```python
from build123d import *

# Parameters (mm, degrees)
SKETCH1_W           = 40.64
SKETCH1_H           = 40.64
BOSS_EXTRUDE1_DEPTH = 5
CUT_EXTRUDE1_REACH  = 7
SKETCH2_R           = 3.085
CHAMFER1_SIZE       = 2.5
SKETCH3_R           = 11.5
CUT_EXTRUDE2_DEPTH  = 1.6
SKETCH7_R           = 0.8
CUT_EXTRUDE6_DEPTH  = 4.4
CUT_EXTRUDE7_DEPTH  = 1.6


with BuildPart() as part:
    # Sketch1 → Boss-Extrude1 (new body)
    with BuildSketch(Plane(origin=(0, 0, 0), x_dir=(1, 0, 0), z_dir=(0, 1, 0))):
        Rectangle(SKETCH1_W, SKETCH1_H)
    extrude(amount=BOSS_EXTRUDE1_DEPTH)

    # Sketch2 → Cut-Extrude1 (cut, up to next)
    with BuildSketch(Plane(origin=(0, 5, 0), x_dir=(1, 0, 0), z_dir=(0, 1, 0)), mode=Mode.PRIVATE) as cut_extrude1_sk1:
        with Locations((-15, 15)):
            Circle(SKETCH2_R)
    cut_extrude1_tool1 = extrude(cut_extrude1_sk1.sketch, amount=-CUT_EXTRUDE1_REACH, mode=Mode.PRIVATE) & part.part
    add(cut_extrude1_tool1.solids().sort_by_distance((-15, 5, -15))[0], mode=Mode.SUBTRACT)
    # Sketch2 → Cut-Extrude1 (cut, up to next)
    with BuildSketch(Plane(origin=(0, 5, 0), x_dir=(1, 0, 0), z_dir=(0, 1, 0)), mode=Mode.PRIVATE) as cut_extrude1_sk2:
        with Locations((15, 15)):
            Circle(SKETCH2_R)
    cut_extrude1_tool2 = extrude(cut_extrude1_sk2.sketch, amount=-CUT_EXTRUDE1_REACH, mode=Mode.PRIVATE) & part.part
    add(cut_extrude1_tool2.solids().sort_by_distance((15, 5, -15))[0], mode=Mode.SUBTRACT)
    # Sketch2 → Cut-Extrude1 (cut, up to next)
    with BuildSketch(Plane(origin=(0, 5, 0), x_dir=(1, 0, 0), z_dir=(0, 1, 0)), mode=Mode.PRIVATE) as cut_extrude1_sk3:
        with Locations((15, -15)):
            Circle(SKETCH2_R)
    cut_extrude1_tool3 = extrude(cut_extrude1_sk3.sketch, amount=-CUT_EXTRUDE1_REACH, mode=Mode.PRIVATE) & part.part
    add(cut_extrude1_tool3.solids().sort_by_distance((15, 5, 15))[0], mode=Mode.SUBTRACT)
    # Sketch2 → Cut-Extrude1 (cut, up to next)
    with BuildSketch(Plane(origin=(0, 5, 0), x_dir=(1, 0, 0), z_dir=(0, 1, 0)), mode=Mode.PRIVATE) as cut_extrude1_sk4:
        with Locations((-15, -15)):
            Circle(SKETCH2_R)
    cut_extrude1_tool4 = extrude(cut_extrude1_sk4.sketch, amount=-CUT_EXTRUDE1_REACH, mode=Mode.PRIVATE) & part.part
    add(cut_extrude1_tool4.solids().sort_by_distance((-15, 5, 15))[0], mode=Mode.SUBTRACT)

    # Chamfer1
    chamfer1_edges = [part.edges().sort_by_distance(p)[0] for p in [
        (20.32, 2.5, 20.32),
        (-20.32, 2.5, 20.32),
        (-20.32, 2.5, -20.32),
        (20.32, 2.5, -20.32),
    ]]
    chamfer(chamfer1_edges, length=CHAMFER1_SIZE)

    # Sketch3 → Cut-Extrude2 (cut)
    with BuildSketch(Plane(origin=(0, 5, 0), x_dir=(1, 0, 0), z_dir=(0, 1, 0))):
        Circle(SKETCH3_R)
    extrude(amount=-CUT_EXTRUDE2_DEPTH, mode=Mode.SUBTRACT)

    # Sketch7 → Cut-Extrude6 (cut, through all)
    with BuildSketch(Plane(origin=(0, 3.4, 0), x_dir=(1, 0, 0), z_dir=(0, 1, 0))):
        with Locations((-8.243053696, -4.727309167)):
            Circle(SKETCH7_R)
        with Locations((8.243053696, 4.727309167)):
            Circle(SKETCH7_R)
    extrude(amount=-CUT_EXTRUDE6_DEPTH, mode=Mode.SUBTRACT)

    # Sketch8 → Cut-Extrude7 (cut)
    with BuildSketch(Plane(origin=(0, 5, 0), x_dir=(1, 0, 0), z_dir=(0, 1, 0))):
        with BuildLine():
            ThreePointArc((2.886406189, -11.131875822), (-0.850588117, -11.468500332), (-4.497034553, -10.584265692))
            Line((-4.497034553, -10.584265692), (2.32, -20.32))
            Line((2.32, -20.32), (9.32, -20.32))
            Line((9.32, -20.32), (2.886406189, -11.131875822))
        make_face()
    extrude(amount=-CUT_EXTRUDE7_DEPTH, mode=Mode.SUBTRACT)


solid = part.part
```
Input: part model. Units: mm. Frame: model coordinates. A direction names the side the tool comes from. Coordinates: 2 decimals unless noted, no trailing zeros. Loops run counter-clockwise (first coordinate to the right, second up) from the corner with the lowest first, then second, coordinate; pieces in that order, holes last. Notation, with made-up numbers: (64.25, 58) -> (102.25, 58) arc R26 ccw to (102.25, 77) -> close; hole circle Ø11 at (-25, 6.25). An arc over 180 degrees is marked (long way). Use a Markdown table: item, result.
1) Pull-direction query (X, two-part tool) for faces 4 (the flat face through (0, 0, 0)), 5 (the flat face through (19.09, 2.47, 19.05)), 6 (the flat face through (-19.05, 2.47, 19.09)), 7 (the cylindrical face through (9.006, 1.724, -4.968)); classes: released by +X, released by -X, zero draft, split by the parting line, or undercut.
Results found:
| item | result |
|---|---|
| face 4 | zero draft |
| face 5 | released by +X |
| face 6 | released by -X |
| face 7 | undercut |
2) Cut plane C-C (z = 0). Return the cut outline in (x, y).
Results found:
| item | result |
|---|---|
| outline | (-20.32, 0) -> (20.32, 0) -> (20.32, 5) -> (11.5, 5) -> (11.5, 3.4) -> (-11.5, 3.4) -> (-11.5, 5) -> (-20.32, 5) -> close |
3) Material intervals for line 1 along X through (y, z) = (2.8, 15) (3 decimals); line 2 along X through (y, z) = (3.85, 15) (3 decimals), sorted ascending. Write a range as from..to.
Results found:
| item | result |
|---|---|
| line 1 | x = -20.32..-18.085, -11.915..11.915, 18.085..20.32 |
| line 2 | x = -20.32..-18.085, -11.915..-1.405, 5.595..11.915, 18.085..20.32 |
4) Access query for faces 1 (the flat face through (6.15, 4.21, 15.79)), 2 (the flat face through (-19.05, 2.47, -19.09)), 3 (the flat face through (0, 3.4, 1)). Directions: +Z, -Z, +X, -X, +Y, -Y. A direction counts if a zero-diameter tool reaches every point of the face in a straight line with its end or side. Return the directions, or none.
Results found:
| item | result |
|---|---|
| face 1 | +Z, +Y |
| face 2 | -Z, -X, +Y, -Y |
| face 3 | +Y |
5) Cut plane A-A (z = -15). Return the cut outline in (x, y) (3 decimals), then the cut area to 4 significant figures.
Results found:
| item | result |
|---|---|
| outline | (-20.32, 0) -> (-18.085, 0) -> (-18.085, 5) -> (-20.32, 5) -> close; (-11.915, 0) -> (11.915, 0) -> (11.915, 5) -> (-11.915, 5) -> close; (18.085, 0) -> (20.32, 0) -> (20.32, 5) -> (18.085, 5) -> close |
| area | 141.5 mm2 |
6) Cut plane D-D (x = 0). Return the cut outline in (y, z).
Results found:
| item | result |
|---|---|
| outline | (0, -20.32) -> (5, -20.32) -> (5, -11.5) -> (3.4, -11.5) -> (3.4, 17.01) -> (5, 17.01) -> (5, 20.32) -> (0, 20.32) -> close |
7) Cut plane B-B (x = -15). Return the cut outline in (y, z) (3 decimals).
Results found:
| item | result |
|---|---|
| outline | (0, -20.32) -> (5, -20.32) -> (5, -18.085) -> (0, -18.085) -> close; (0, -11.915) -> (5, -11.915) -> (5, 11.915) -> (0, 11.915) -> close; (0, 18.085) -> (5, 18.085) -> (5, 20.32) -> (0, 20.32) -> close |
